Study the drawing (mm; zero at the part's minimum x, y, z) and answer. A direction names the side the tool comes from. Round coordinates to 2 decimals unless told otherwise and drop trailing zeros. Loops run counter-clockwise (first coordinate to the right, second up) from the corner with the lowest first, then second, coordinate; pieces in that order, holes last. Notation, with made-up numbers: (17, 64.5) -> (75, 64.5) arc R25 ccw to (75, 101.5) -> close; hole circle Ø11 at (27, 57). An arc over 180 degrees is marked (long way). Answer in a Markdown table with one row per item. Add a question column.
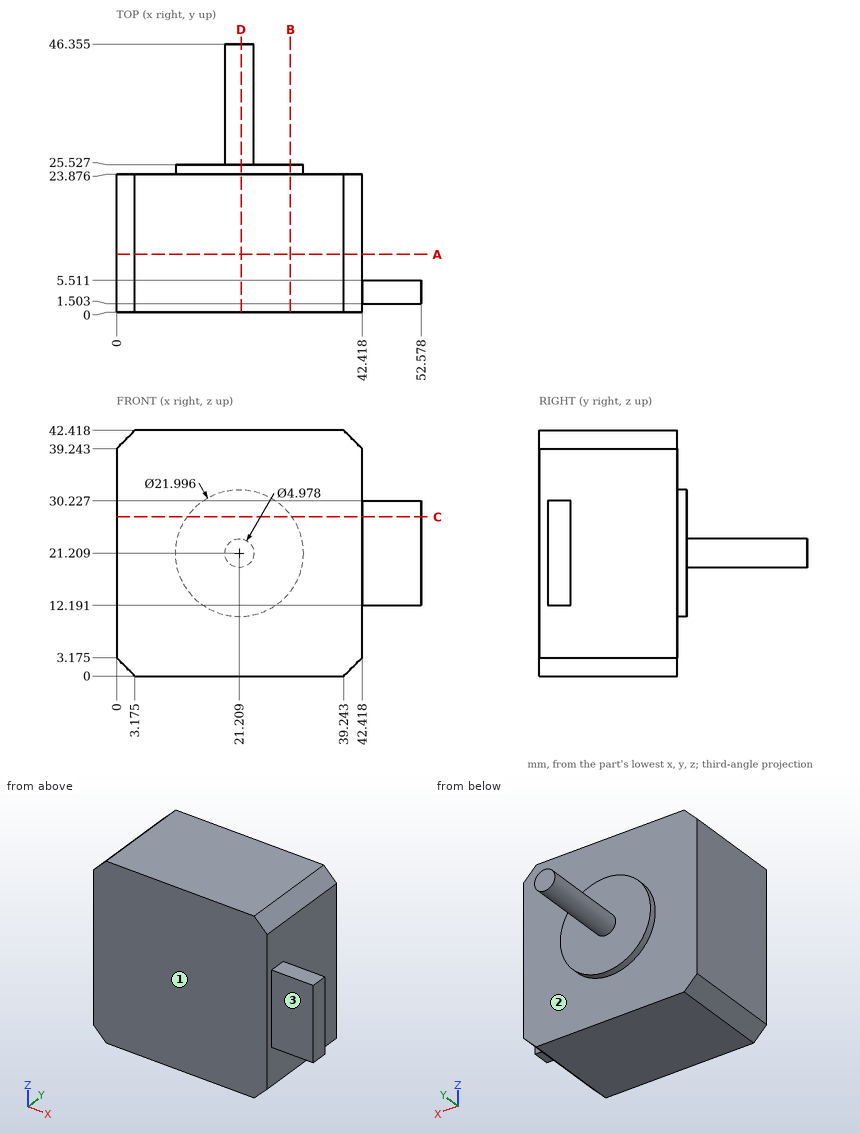
Item 1: Section B-B, the plane x = 30 is taken. Write down the section's boundary in (y, z).
Item 2: Section D-D, the plane x = 21.5 is taken. Write down the section's boundary in (y, z) (1 decimal), and give its area (3 significant figures).
Item 3: For the marked faces 1, 2 and 3, determine the directions among +Z, -Z, +X, -X, +Y, -Y from which every point of the face is accessible in a straight line to the end or side of a thin tool.
Item 4: Consider L1, parallel to Y at x = 41, z = 7.5; L2, parallel to X at y = 13, z = 35; L3, parallel to Y at x = 19, z = 18. Determine where each line is inside the solid, lowest interval first. Write a range as from..to.
Item 5: Section A-A, the plane y = 10 is taken. Write down the section's boundary in (x, z) (1 decimal).
Item 6: Section C-C, the plane z = 27.5 is taken. Write down the section's boundary in (x, y), and give its area (3 significant figures).
Item 7: Flat-ended cylindrical pins translate along their axes: P1, Ø12.5, axis at x = 12.5, z = 16.5, coming from the +Y side; P2, Ø5, axis at x = 11.5, y = 27.5, coming from the +Z side; P3, Ø5, axis at x = 50, z = 18.5, coming from the -Y side; P4, Ø5, axis at x = 32.5, y = 29.5, coming from the -Z side. Find the tip coordinate at first contact, or state that the pin passes through.
Here are the results:
| question | item | result |
|---|---|---|
| 1 | outline | (0, 0) -> (23.88, 0) -> (23.88, 14.6) -> (25.53, 14.6) -> (25.53, 27.82) -> (23.88, 27.82) -> (23.88, 42.42) -> (0, 42.42) -> close |
| 2 | outline | (0, 0) -> (23.9, 0) -> (23.9, 10.2) -> (25.5, 10.2) -> (25.5, 18.7) -> (46.4, 18.7) -> (46.4, 23.7) -> (25.5, 23.7) -> (25.5, 32.2) -> (23.9, 32.2) -> (23.9, 42.4) -> (0, 42.4) -> close |
| 2 | area | 1,150 mm² |
| 3 | face 1 | +Z, -Z, +X, -X, -Y |
| 3 | face 2 | +Y |
| 3 | face 3 | +Z, -Z, +X, -Y |
| 4 | L1 | y = 0..23.88 |
| 4 | L2 | x = 0..42.42 |
| 4 | L3 | y = 0..25.53 |
| 5 | outline | (0, 3.2) -> (3.2, 0) -> (39.2, 0) -> (42.4, 3.2) -> (42.4, 39.2) -> (39.2, 42.4) -> (3.2, 42.4) -> (0, 39.2) -> close |
| 6 | outline | (0, 0) -> (42.42, 0) -> (42.42, 1.5) -> (52.58, 1.5) -> (52.58, 5.51) -> (42.42, 5.51) -> (42.42, 23.88) -> (30.23, 23.88) -> (30.23, 25.53) -> (12.19, 25.53) -> (12.19, 23.88) -> (0, 23.88) -> close |
| 6 | area | 1,080 mm² |
| 7 | P1 | stops at y = 25.53 |
| 7 | P2 | stops at z = 28.57 |
| 7 | P3 | stops at y = 1.5 |
| 7 | P4 | passes through |
